from build123d import *

# Parameters (mm, degrees)
F1_DEPTH = 63.5
F0_W     = 25.6538060188
F0_H     = 19.05
F2_DEPTH = 25.4
F3_DEPTH = 7.9375
F5_R     = 6.35


with BuildPart() as f1:
    # F0 (on Front) → F1 (new body, symmetric)
    with BuildSketch(Plane.XZ):
        Polygon((22.225, 9.525), (-41.275, 9.525), (-41.275, -9.525), (41.275, -9.525), (41.275, 9.525), align=None)
    extrude(amount=F1_DEPTH, both=True)

    # F0 (on Front) → F2 (join, symmetric)
    with BuildSketch(Plane.XZ):
        with Locations((73.1519030094, 52.4002)):
            Rectangle(F0_W, F0_H)
        with BuildLine():
            Line((22.225, 27.0002), (22.225, 9.525))
            Line((22.225, 9.525), (41.275, 9.525))
            Line((41.275, 9.525), (41.275, 27.0002))
            ThreePointArc((41.275, 27.0002), (45.9246798487, 38.2255201513), (57.15, 42.8752))
            Line((57.15, 42.8752), (60.325, 42.8752))
            Line((60.325, 42.8752), (60.325, 61.9252))
            Line((60.325, 61.9252), (57.15, 61.9252))
            ThreePointArc((57.15, 61.9252), (32.4542956671, 51.6959043329), (22.225, 27.0002))
        make_face()
    extrude(amount=F2_DEPTH, both=True)

    # F0 (on Front) → F3 (join, symmetric)
    with BuildSketch(Plane.XZ):
        with BuildLine():
            add(Edge.make_bspline(
                [(-41.275, 9.525), (-41.1863140762, 29.6085979789), (0, 67.188732326), (57.15, 61.9252)],
                knots=[0, 0, 0, 0, 111.5045361635, 111.5045361635, 111.5045361635, 111.5045361635], degree=3))
            Line((-41.275, 9.525), (22.225, 9.525))
            Line((22.225, 9.525), (22.225, 27.0002))
            ThreePointArc((22.225, 27.0002), (32.4542956671, 51.6959043329), (57.15, 61.9252))
        make_face()
    extrude(amount=F3_DEPTH, both=True)

    # F0 (on Front) → F4 (revolve)
    with BuildSketch(Plane.XZ):
        Polygon((85.9788060188, 66.675), (85.9788060188, 61.9252), (85.9788060188, 42.8752), (85.9788060188, 38.1), (111.125, 38.1), (111.125, 66.675), align=None)
    revolve(axis=Axis((85.9788060188, 0, 54.7751), (0, 0, -1)))

    # F5
    f5_edges = [f1.edges().sort_by_distance(p)[0] for p in [
        (41.275, -63.5, 0),
        (-41.275, -63.5, 0),
        (41.275, 63.5, 0),
        (-41.275, 63.5, 0),
    ]]
    fillet(f5_edges, radius=F5_R)


solid = f1.part
Input: part model. Units: mm. Frame: model coordinates. A direction names the side the tool comes from. Give positions to 0.01 mm unless a question says otherwise; leave off trailing zeros. Order: outer loops, then holes, each group sorted by start corner. A loop starts at its lowest first (then second) coordinate and runs counter-clockwise, first axis right, second up.
Q1. Section D-D on y = 20. Output: boundary loops of the cut face in (x, z) (3 decimals).
Checked values:
outline: (-41.275, -9.525) - (41.275, -9.525) - (41.275, 27) arc R15.875 cw to (57.15, 42.875) - (70.736, 42.875) - (70.736, 38.1) - (101.221, 38.1) - (101.221, 66.675) - (70.736, 66.675) - (70.736, 61.925) - (57.15, 61.925) arc R34.925 ccw to (22.225, 27) - (22.225, 9.525) - (-41.275, 9.525) - close
Q2. Ray query, probe 1 along Z at (x, y) = (-31.5, 38.5) (3 decimals); probe 2 along Y at (x, z) = (29.5, 46); probe 3 along Z at (x, y) = (85, 16) (3 decimals). Return the intervals inside material, ascending.
Checked values:
probe 1: z = -9.525 to 9.525
probe 2: y = -25.4 to 25.4
probe 3: z = 38.1 to 66.675
Q3. Section C-C on y = -23. Output: boundary loops of the cut face in (x, z) (3 decimals), and give its area (3 significant figures).
Checked values:
outline: (-41.275, -9.525) - (41.275, -9.525) - (41.275, 27) arc R15.875 cw to (57.15, 42.875) - (75.814, 42.875) - (75.814, 38.1) - (96.144, 38.1) - (96.144, 66.675) - (75.814, 66.675) - (75.814, 61.925) - (57.15, 61.925) arc R34.925 ccw to (22.225, 27) - (22.225, 9.525) - (-41.275, 9.525) - close
area: 3,600 mm2
Q4. Section A-A on z = 2. Output: boundary loops of the cut face in (x, y) (3 decimals).
Checked values:
outline: (-41.275, -57.15) arc R6.35 ccw to (-34.925, -63.5) - (34.925, -63.5) arc R6.35 ccw to (41.275, -57.15) - (41.275, 57.15) arc R6.35 ccw to (34.925, 63.5) - (-34.925, 63.5) arc R6.35 ccw to (-41.275, 57.15) - close
Q5. Section B-B on x = 80. Output: boundary loops of the cut face in (y, z) (3 decimals).
Checked values:
outline: (-25.4, 42.875) - (-24.425, 42.875) - (-24.425, 38.1) - (24.425, 38.1) - (24.425, 42.875) - (25.4, 42.875) - (25.4, 61.925) - (24.425, 61.925) - (24.425, 66.675) - (-24.425, 66.675) - (-24.425, 61.925) - (-25.4, 61.925) - close
Q6. Contact query for flat-ended pins moving along their axis: pin 1 Ø8.5 at (x, y) = (66, 8.5) entering from -Z; pin 2 Ø6 at (y, z) = (26, 50.5) entering from -X; pin 3 Ø8.5 at (y, z) = (12.5, 16.5) entering from -X (3 decimals). Output: stop coordinate, or through.
Checked values:
pin 1: stops at z = 38.1
pin 2: stops at x = 28.92
pin 3: stops at x = 22.225
Q7. Draft query along X for faces 1 (the cylindrical face through (45.8, -0.4, 38.1)), 2 (the flat face through (41.275, -1, 4)), 3 (the flat face through (-1, -1, -9.525)). Return one class per face: +X half, -X half, draft (parallel to the pull), parting line (faces both ways), or undercut.
Checked values:
face 1: undercut
face 2: +X half
face 3: draft
Q8. Set-up query: faces 4 (the flat face through (-2, -7.938, 32)), 5 (the cylindrical face through (32.73, 16.55, 51.97)), 6 (the flat face through (86, 0, 38.1)). Return all of +Z, -Z, +X, -X, +Y, -Y with unobstructed straight access to the full face (end or side cutting, diameter ignored); none if empty.
Checked values:
face 4: +Z, -X, -Y
face 5: +Z, -X, +Y
face 6: -Z, +X, +Y, -Y
